from build123d import *

# Parameters (mm, degrees)
SKETCH1_W           = 160
SKETCH1_H           = 18
BOSS_EXTRUDE1_DEPTH = 15
CUT_EXTRUDE1_DEPTH  = 161
SKETCH3_W           = 10
SKETCH3_H           = 10
BOSS_EXTRUDE2_DEPTH = 10


with BuildPart() as part:
    # Sketch1 → Boss-Extrude1 (new body)
    with BuildSketch(Plane.XY):
        with Locations((415.087037167, 89.382420628)):
            Rectangle(SKETCH1_W, SKETCH1_H)
    extrude(amount=BOSS_EXTRUDE1_DEPTH)

    # Sketch2 → Cut-Extrude1 (cut, through all)
    with BuildSketch(Plane(origin=(495.087037167, 0, 0), x_dir=(0, 0, -1), z_dir=(1, 0, 0))):
        Polygon((-12.5, 98.382420628), (-11.056624327, 95.882420628), (-6.056624327, 95.882420628), (-4.613248654, 98.382420628), align=None)
        Polygon((-4.613248654, 80.382420628), (-12.5, 80.382420628), (-11.056624327, 82.882420628), (-6.056624327, 82.882420628), align=None)
    extrude(amount=-CUT_EXTRUDE1_DEPTH, mode=Mode.SUBTRACT)

    # Sketch3 → Boss-Extrude2 (add)
    with BuildSketch(Plane(origin=(0, 0, 0), x_dir=(-1, 0, 0), z_dir=(0, 0, -1))):
        with Locations((-415.087037167, 89.382420628)):
            Rectangle(SKETCH3_W, SKETCH3_H)
    extrude(amount=BOSS_EXTRUDE2_DEPTH)


solid = part.part
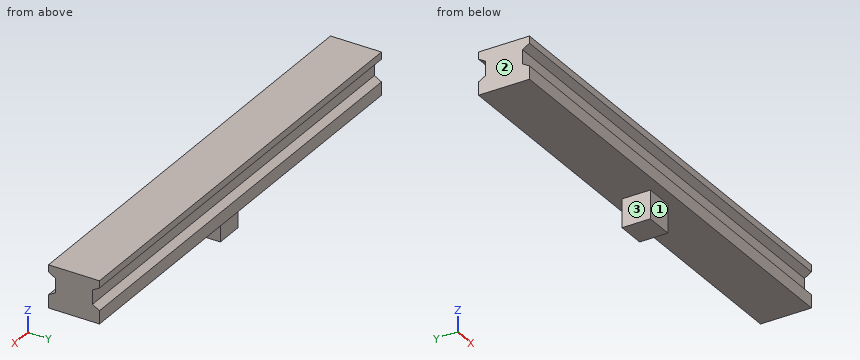
Can you work these out from the model? Positions are in its coordinate system, mm. Face numbers are marked on the shaded views. A direction names the side the tool comes from. Round coordinates to 2 decimals unless told otherwise and drop trailing zeros. Write each loop counter-clockwise with the first axis right and the second up, starting at its lowest first coordinate (ties: lowest second). Pieces come first, ordered by that corner, then holes. Notation, with made-up numbers: (84.5, 34.25) -> (139.5, 34.25) arc R14 ccw to (139.5, 47.25) -> close; hole circle Ø7 at (44.25, 63.25). An arc over 180 degrees is marked (long way). Use one line per item in the form item = value. Start each with the question number.
Q1. I'm going to push flat-ended pins straight in: P1, Ø5, axis at y = 89.5, z = -3.5, coming from the -X side; P2, Ø2.5, axis at x = 418.5, z = 9.5, coming from the +Y side; P3, Ø1, axis at x = 355, y = 88.5, coming from the -Z side; P4, Ø1, axis at y = 82.5, z = -2, coming from the +X side. Where does each tip first touch, or does it pass through?
Q2. Imagine slicing it at B-B (y = 93). Please give me the cut outline in (x, z), then the cut area to 3 significant figures.
Q3. Imagine slicing it at D-D (z = -2.5). Please give me the cut outline in (x, y), then the cut area to 3 significant figures.
Q4. Which directions (+Z, -Z, +X, -X, +Y, -Y) give clear straight access to the entire face, cutting with the end or side of a thin tool? Please do the marked faces 1, 2 and 3.
Q5. Imagine slicing it at C-C (z = 8.75). Please give me the cut outline in (x, y).
Q6. Imagine slicing it at A-A (x = 394). Please give me the cut outline in (y, z).
Q7. If I drill on probe 1 along Z at (x, y) = (375.5, 83.25); probe 2 along Z at (x, y) = (446, 97.75); probe 3 along Y at (x, z) = (413.5, -3.25), over which ranges is the centre line in solid material (lowest first)? Write a range as [from, to].
Worked out:
q1.P1 = 410.09
q1.P2 = 95.88
q1.P3 = 0
q1.P4 = through
q2.outline = (335.09, 0) -> (410.09, 0) -> (410.09, -10) -> (420.09, -10) -> (420.09, 0) -> (495.09, 0) -> (495.09, 15) -> (335.09, 15) -> close
q2.area = 2,500 mm^2
q3.outline = (410.09, 84.38) -> (420.09, 84.38) -> (420.09, 94.38) -> (410.09, 94.38) -> close
q3.area = 100 mm^2
q4.face_1 = -Z, +X, -X, -Y
q4.face_2 = +Z, -Z, -X, +Y, -Y
q4.face_3 = -Z, -X, +Y, -Y
q5.outline = (335.09, 82.88) -> (495.09, 82.88) -> (495.09, 95.88) -> (335.09, 95.88) -> close
q6.outline = (80.38, 0) -> (98.38, 0) -> (98.38, 4.61) -> (95.88, 6.06) -> (95.88, 11.06) -> (98.38, 12.5) -> (98.38, 15) -> (80.38, 15) -> (80.38, 12.5) -> (82.88, 11.06) -> (82.88, 6.06) -> (80.38, 4.61) -> close
q7.probe_1 = [0, 15]
q7.probe_2 = [0, 4.98], [12.13, 15]
q7.probe_3 = [84.38, 94.38]
